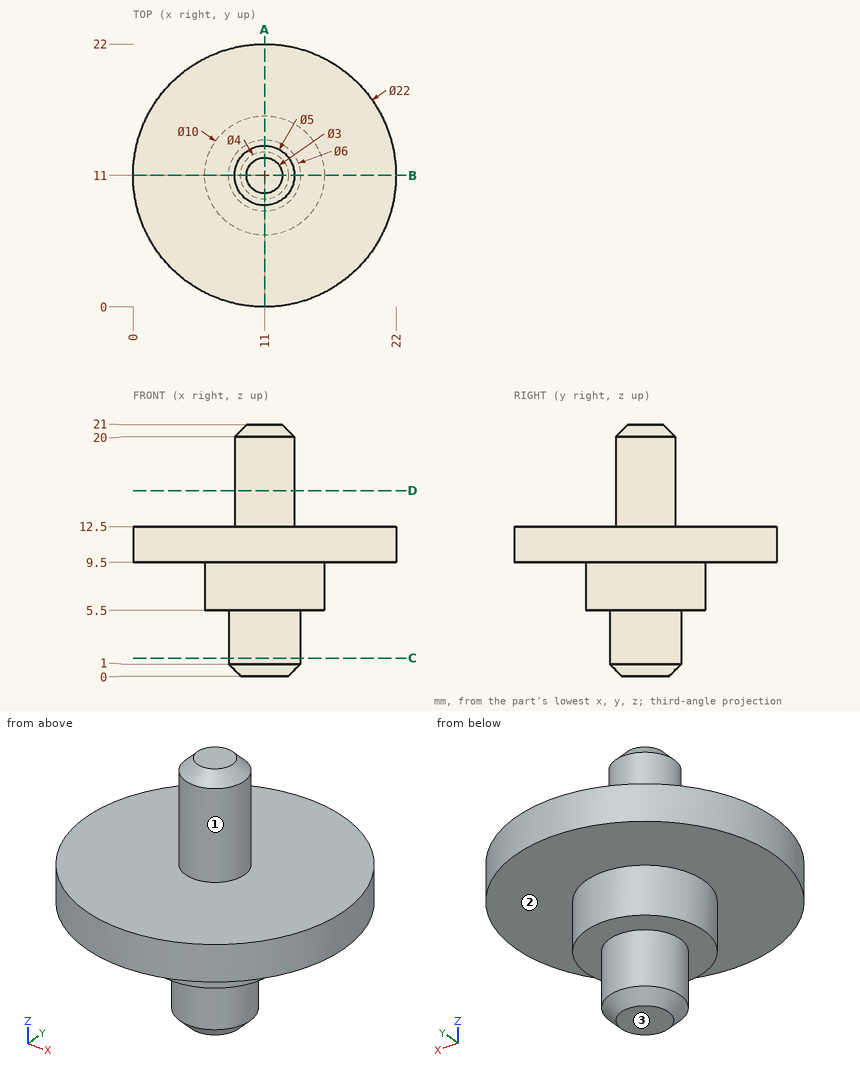
The drawing under review shows one solid part. Ordinate dimensions are in mm from its lowest x, y, z. A direction names the side the tool comes from. Give positions to 0.01 mm unless a question says otherwise; leave off trailing zeros. Order: outer loops, then holes, each group sorted by start corner. A loop starts at its lowest first (then second) coordinate and runs counter-clockwise, first axis right, second up. Notation, with made-up numbers: (29.5, 66) - (54.5, 66) arc R18 cw to (54.5, 73) - close; hole circle Ø5 at (28, -12). An arc over 180 degrees is marked (long way). Answer as a JSON object with one key per item and string values. Group by question number.
Item 1: Take a section at C-C on z = 1.5. Give the boundary of the cut face in (x, y), and give its area (3 significant figures).
Item 2: Take a section at D-D on z = 15.5. Give the boundary of the cut face in (x, y).
Item 3: Wall thickness on line 1 along Z through (x, y) = (18, 17.25); line 2 along X through (y, z) = (10.75, 9); line 3 along Y through (x, z) = (11, 13): over which ranges is each line inside the solid? List them lowest first.
Item 4: Take a section at A-A on x = 11. Give the boundary of the cut face in (y, z).
Item 5: Machinability: for the marked faces 1, 2 and 3, which of the approach directions +Z, -Z, +X, -X, +Y, -Y give a long, thin tool a straight path to every point of the face, cutting with its end or side? Answer none if there is none.
Item 6: Clearance check with flat-ended pins moving along their axes: pin 1 Ø6.5 at (x, y) = (15.5, 8) entering from +Z; pin 2 Ø1 at (x, y) = (19.5, 16) entering from +Z; pin 3 Ø1 at (y, z) = (13, 3) entering from +X; pin 4 Ø8 at (x, y) = (12.5, 10) entering from -Z. State where each tip first meets the part, or that it passes through.
Reported:
{
 "1": {"outline": "circle Ø6 at (11, 11)", "area": "28.3 mm^2"},
 "2": {"outline": "circle Ø5 at (11, 11)"},
 "3": {"line 1": "9.5 to 12.5", "line 2": "6.01 to 15.99", "line 3": "8.5 to 13.5"},
 "4": {"outline": "(0, 9.5) - (6, 9.5) - (6, 5.5) - (8, 5.5) - (8, 1) - (9, 0) - (13, 0) - (14, 1) - (14, 5.5) - (16, 5.5) - (16, 9.5) - (22, 9.5) - (22, 12.5) - (13.5, 12.5) - (13.5, 20) - (12.5, 21) - (9.5, 21) - (8.5, 20) - (8.5, 12.5) - (0, 12.5) - close"},
 "5": {"face 1": "+Z", "face 2": "-Z", "face 3": "-Z, +X, -X, +Y, -Y"},
 "6": {"pin 1": "z = 20.34", "pin 2": "z = 12.5", "pin 3": "x = 13.6", "pin 4": "z = 0"}
}
